The listing builds one solid part. Answer for the finished solid, in the listing's coordinates (mm). Face numbers are marked on the shaded views. A direction names the side the tool comes from. Give positions to 0.01 mm unless a question says otherwise; leave off trailing zeros. Loops run counter-clockwise (first coordinate to the right, second up) from the corner with the lowest first, then second, coordinate; pieces in that order, holes last.
Item 1: A tool of negligible diameter and unlimited length cuts with its end or side. For the marked faces 3 and 4, from which of +Z, -Z, +X, -X, +Y, -Y can it reach the whole face along a straight path? Write none if from no direction.
Item 2: The mould has two halves that part along X. Classify the marked faces 1 and 2: pulls with the +X half, pulls with the -X half, needs draft (parallel to the pull), parting line crosses it, or undercut.
Item 3: Section A-A, the plane y = -1.35 is taken. Give the vertices of the cut face in (x, z) (3 decimals), and give its area (3 significant figures).
Item 4: Each of these flat-tipped pins is pushed along its axis until it touches: pin 1 Ø0.8 at (x, z) = (2.5, 0.5) entering from +Y; pin 2 Ø0.8 at (x, z) = (2.5, 0.5) entering from -Y; pin 3 Ø1.9 at (x, y) = (0.5, -0.5) entering from -Z; pin 4 Ø1.5 at (x, y) = (2, 2) entering from +Z (3 decimals). Where does it stop, or does it pass through?
Item 5: Section C-C, the plane x = 0 is taken. Give the vertices of the cut face in (y, z).
Item 6: Consider line 1 along Y through (x, z) = (2.25, 0.9); line 2 along X through (y, z) = (-1.55, 0.25); line 3 along Z through (x, y) = (-1, 0.05). Determine where each line is inside the solid, lowest interval first.
Item 7: Section B-B, the plane z = 0.35 is taken. Give the vertices of the cut face in (x, y).
from build123d import *

# Parameters (mm, degrees)
PAD_DEPTH    = 2.35
CHAMFER_SIZE = 0.25
POCKET_DEPTH = 0.2
PAD003_DEPTH = 0.35
PAD002_DEPTH = 0.35
SKETCH005_W  = 0.4
SKETCH005_H  = 4.4
PAD004_DEPTH = 0.075


with BuildPart() as pocket:
    # Sketch → Pad (new body, symmetric)
    with BuildSketch(Plane.XZ):
        Polygon((-1.9, 0.1), (1.9, 0.1), (1.95, 0.85), (1.9, 1.6), (-1.9, 1.6), (-1.95, 0.85), align=None)
    extrude(amount=PAD_DEPTH, both=True)

    # Chamfer
    chamfer_edges = [pocket.edges().sort_by_distance(p)[0] for p in [
        (1.9, 0, 1.6),
    ]]
    chamfer(chamfer_edges, length=CHAMFER_SIZE)

    # Sketch004 → Pocket (cut)
    with BuildSketch(Plane(origin=(0, 0, 1.6), x_dir=(-1, 0, 0), z_dir=(0, 0, 1))):
        with BuildLine():
            ThreePointArc((0.5, -1.85), (0, -1.35), (-0.5, -1.85))
            Line((-0.5, -1.85), (-0.5, -2.35))
            Line((-0.5, -2.35), (0.5, -2.35))
            Line((0.5, -2.35), (0.5, -1.85))
        make_face()
    extrude(amount=-POCKET_DEPTH, mode=Mode.SUBTRACT)


with BuildPart() as pad003:
    # Sketch003 → Pad003 (new body, symmetric)
    with BuildSketch(Plane.XZ.offset(-1.27)):
        Polygon((-3.25, 0), (-2.55, 0), (-2.3, 0.75), (2.3, 0.75), (2.55, 0), (3.25, 0), (3.25, 0.2), (2.65, 0.2), (2.4, 0.95), (-2.4, 0.95), (-2.65, 0.2), (-3.25, 0.2), align=None)
    extrude(amount=PAD003_DEPTH, both=True)


with BuildPart() as pad002:
    # Sketch002 → Pad002 (new body, symmetric)
    with BuildSketch(Plane.XZ.offset(1.27)):
        Polygon((-3.25, 0), (-2.55, 0), (-2.3, 0.75), (2.3, 0.75), (2.55, 0), (3.25, 0), (3.25, 0.2), (2.65, 0.2), (2.4, 0.95), (-2.4, 0.95), (-2.65, 0.2), (-3.25, 0.2), align=None)
    extrude(amount=PAD002_DEPTH, both=True)


with BuildPart() as to_269aa:
    # Sketch005 → Pad004 (new body)
    with BuildSketch(Plane.XY.offset(1.55)):
        with Locations((1.3, 0)):
            Rectangle(SKETCH005_W, SKETCH005_H)
    extrude(amount=PAD004_DEPTH)

    add(pocket.part)
    add(pad003.part)
    add(pad002.part)


solid = to_269aa.part
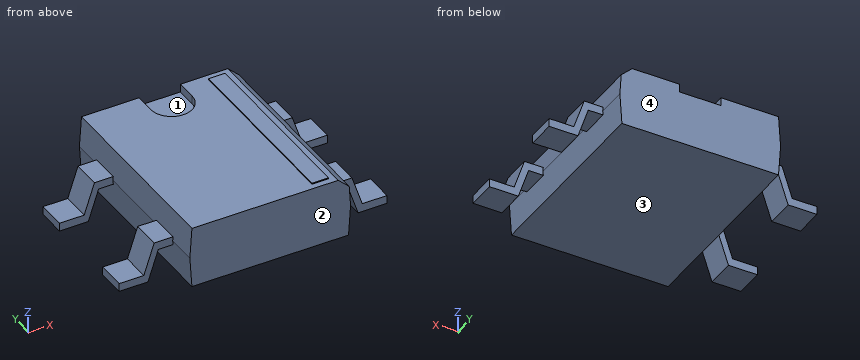
Worked answers:
1. face 3: -Z, +Y, -Y
1. face 4: +Z, -Z, +X, -X, +Y
2. face 1: undercut
2. face 2: needs draft
3. outline: (-3.25, 0) - (-2.55, 0) - (-2.3, 0.75) - (-1.943, 0.75) - (-1.9, 0.1) - (1.9, 0.1) - (1.943, 0.75) - (2.3, 0.75) - (2.55, 0) - (3.25, 0) - (3.25, 0.2) - (2.65, 0.2) - (2.4, 0.95) - (1.943, 0.95) - (1.917, 1.351) - (1.65, 1.6) - (1.5, 1.6) - (1.5, 1.625) - (1.1, 1.625) - (1.1, 1.6) - (-1.9, 1.6) - (-1.943, 0.95) - (-2.4, 0.95) - (-2.65, 0.2) - (-3.25, 0.2) - close
3. area: 6.43 mm2
4. pin 1: stops at y = 1.62
4. pin 2: stops at y = -1.62
4. pin 3: stops at z = 0.1
4. pin 4: stops at z = 1.625
5. outline: (-2.35, 0.1) - (2.35, 0.1) - (2.35, 1.4) - (1.35, 1.4) - (1.35, 1.6) - (-2.35, 1.6) - close
6. line 1: y = -1.62 to -0.92, 0.92 to 1.62
6. line 2: x = -2.63 to -2.47, -1.91 to 1.91, 2.47 to 2.63
6. line 3: z = 0.1 to 1.6
7. outline: (-2.6, -1.62) - (-2.43, -1.62) - (-2.43, -0.92) - (-2.6, -0.92) - close; (-2.6, 0.92) - (-2.43, 0.92) - (-2.43, 1.62) - (-2.6, 1.62) - close; (-1.92, -2.35) - (1.92, -2.35) - (1.92, 2.35) - (-1.92, 2.35) - close; (2.43, -1.62) - (2.6, -1.62) - (2.6, -0.92) - (2.43, -0.92) - close; (2.43, 0.92) - (2.6, 0.92) - (2.6, 1.62) - (2.43, 1.62) - close
